Part model, mm, in its own coordinate system. A direction names the side the tool comes from. Coordinates: 2 decimals unless noted, no trailing zeros. Loops run counter-clockwise (first coordinate to the right, second up) from the corner with the lowest first, then second, coordinate; pieces in that order, holes last. Notation, with made-up numbers: (-27.75, 43.5) - (5.25, 43.5) arc R18 ccw to (5.25, 62.5) - close; hole circle Ø11 at (75.5, 13.5). An arc over 180 degrees is marked (long way). Answer as CSV lines item,"result".
from build123d import *

# Parameters (mm, degrees)
SKETCH007_R     = 3.65
PAD005_DEPTH    = 55
SKETCH008_R     = 1.5
SKETCH008_R_2   = 3.7
PAD006_DEPTH    = 5
PAD007_DEPTH    = 2.5
SKETCH010_W     = 40
SKETCH010_H     = 45
POCKET001_DEPTH = 6.5
CHAMFER_SIZE    = 5.99


with BuildPart() as part:
    # Sketch007 → Pad005 (new body)
    with BuildSketch(Plane.XY):
        with BuildLine():
            ThreePointArc((0, -15), (8.5, -23.5), (17, -15))
            Line((17, 0), (17, -15))
            Line((0, 0), (17, 0))
            Line((0, -15), (0, 0))
        make_face()
        with Locations((8.5, -15)):
            Circle(SKETCH007_R, mode=Mode.SUBTRACT)
    extrude(amount=-PAD005_DEPTH)

    # Sketch008 → Pad006 (join)
    with BuildSketch(Plane.XY):
        with BuildLine():
            Line((23.5, 0), (23.5, 50))
            Line((23.5, 50), (-6.5, 50))
            Line((-6.5, 50), (-6.5, 0))
            Line((0, -15), (-6.5, 0))
            ThreePointArc((0, -15), (8.5, -23.5), (17, -15))
            Line((17, -15), (23.5, 0))
        make_face()
        with Locations((17.5, 12)):
            Circle(SKETCH008_R, mode=Mode.SUBTRACT)
        with Locations((17.5, 38)):
            Circle(SKETCH008_R, mode=Mode.SUBTRACT)
        with Locations((-1.694422, 38)):
            Circle(SKETCH008_R, mode=Mode.SUBTRACT)
        with Locations((-1.694422, 12)):
            Circle(SKETCH008_R, mode=Mode.SUBTRACT)
        with Locations((8.5, -15)):
            Circle(SKETCH008_R_2, mode=Mode.SUBTRACT)
    extrude(amount=-PAD006_DEPTH)

    # Sketch009 (on DatumPlane) → Pad007 (join, symmetric)
    with BuildSketch(Plane(origin=(8.5, 0, 1), x_dir=(0, 1, 0), z_dir=(1, 0, 0))):
        Polygon((0, -56), (0, -6), (50, -6), (10, -56), align=None)
        Polygon((6, -12), (6, -48), (38, -12), align=None, mode=Mode.SUBTRACT)
    extrude(amount=PAD007_DEPTH, both=True)

    # Sketch010 (on DatumPlane) → Pocket001 (cut, symmetric)
    with BuildSketch(Plane(origin=(8.5, 0, 1), x_dir=(0, 1, 0), z_dir=(1, 0, 0))):
        with Locations((-22, -28.5)):
            Rectangle(SKETCH010_W, SKETCH010_H)
    extrude(amount=POCKET001_DEPTH, both=True, mode=Mode.SUBTRACT)

    # Chamfer
    chamfer_edges = [part.edges().sort_by_distance(p)[0] for p in [
        (6, 0, -30),
        (11, 0, -30),
    ]]
    chamfer(chamfer_edges, length=CHAMFER_SIZE)


with BuildPart() as part_1:
    # Body003 placement: moved
    add(part.part.moved(Location((0, 0, -4))))


solid = part_1.part
Q1. Wall check: L1, parallel to Y at x = 17.5, z = -6.2; L2, parallel to Y at x = 8.5, z = -7.05; L3, parallel to Z at x = 4, y = -20.5. Give the ranges that are in metal, low to high.
Results:
L1,"y = -13.85 to 10.5, 13.5 to 36.5, 39.5 to 50"
L2,"y = -23.5 to -18.65, -11.35 to 50"
L3,"z = -59 to -54, -9 to -4"
Q2. Saw through at B-B (x = 8.5). Give the cut face in (y, z), then the cut area to 3 significant figures.
Results:
outline,"(-23.5, -59) - (-18.65, -59) - (-18.65, -54) - (-23.5, -54) - close; (-23.5, -9) - (-18.65, -9) - (-18.65, -4) - (-23.5, -4) - close; (-11.35, -59) - (10, -59) - (50, -9) - (50, -4) - (-11.35, -4) - (-11.35, -9) - (-2, -9) - (-2, -54) - (-11.35, -54) - close; hole (6, -51) - (38, -15) - (6, -15) - close"
area,"1,430 mm^2"
Q3. Flat gauge pins, fed straight in: pin 1 (6.5 mm diameter, centred on x = 11.5, z = -27.5, fed in from -Y); pin 2 (20.5 mm diameter, centred on y = -13.5, z = -25.5, fed in from +X); pin 3 (12 mm diameter, centred on x = 9.5, y = 33.5, fed in from -Z) (3 decimals); pin 4 (14.5 mm diameter, centred on x = 10, y = -12, fed in from -Z). Where does each tip first touch, or does it go through?
Results:
pin 1,"stops at y = -2"
pin 2,"stops at x = 17"
pin 3,"stops at z = -37.125"
pin 4,"stops at z = -59"
Q4. Two-plate mould, pull along Y, no slides. Class faces 4 (the face through (9, 50, -6)), 5 (the face through (16, 12, -6)), 6 (the face through (-3.205, -7.605, -6.465)), 7 (the face through (8, -7, -59)): released by +Y, released by -Y, zero draft, split by the parting line, or undercut.
Results:
face 4,"released by +Y"
face 5,"undercut"
face 6,"released by -Y"
face 7,"zero draft"
Q5. Which spindle directions (+Z, -Z, +X, -X, +Y, -Y) get a long thin tool onto all of the face, cutting with end or side? Do faces 1 (the face through (9, 22, -33)), 2 (the face through (11, 26.5, -28.3)), 3 (the face through (9, -11, -54)). Say none if no direction does.
Results:
face 1,"+X, -X"
face 2,"-Z, +X, +Y"
face 3,"-Y"
Q6. Saw through at D-D (y = 32). Give the cut face in (x, z).
Results:
outline,"(-6.5, -9) - (6, -9) - (6, -15) - (11, -15) - (11, -9) - (23.5, -9) - (23.5, -4) - (-6.5, -4) - close; (6, -31.5) - (11, -31.5) - (11, -21.75) - (6, -21.75) - close"
Q7. Saw through at C-C (y = -10.5). Give the cut face in (x, z), then the cut area to 4 significant figures.
Results:
outline,"(-1.95, -9) - (0, -9) - (0, -59) - (17, -59) - (17, -9) - (18.95, -9) - (18.95, -4) - (-1.95, -4) - close; hole (2, -54) - (15, -54) - (15, -9) - (2, -9) - close"
area,"369.5 mm^2"
